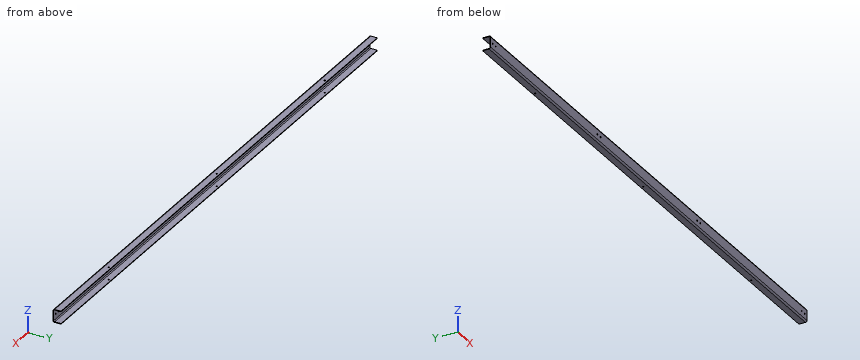
```python
from build123d import *

# Parameters (mm, degrees)
BASE_FLANGE1_DEPTH = 1928.8125
SKETCH2_R          = 2.4511
CUT_EXTRUDE1_DEPTH = 1930.51962345
SKETCH3_R          = 2.4511
CUT_EXTRUDE2_DEPTH = 1930.51962345
FILLET1_R          = 3.175


# Sheet-metal steps are written as plain solids
with BuildPart() as part:
    # Sketch1 → Base-Flange1 (new body)
    with BuildSketch(Plane(origin=(0, 0, 0), x_dir=(0, 0, -1), z_dir=(1, 0, 0))):
        with BuildLine():
            Line((0, 27.432), (0, 5.207))
            ThreePointArc((0, 5.207), (1.52509499, 1.52509499), (5.207, 0))
            Line((5.207, 0), (39.243, 0))
            ThreePointArc((39.243, 0), (42.92490501, 1.52509499), (44.45, 5.207))
            Line((44.45, 5.207), (44.45, 27.432))
            Line((44.45, 27.432), (42.418, 27.432))
            Line((42.418, 27.432), (42.418, 5.207))
            ThreePointArc((42.418, 5.207), (41.48806403, 2.96193597), (39.243, 2.032))
            Line((39.243, 2.032), (5.207, 2.032))
            ThreePointArc((5.207, 2.032), (2.96193597, 2.96193597), (2.032, 5.207))
            Line((2.032, 5.207), (2.032, 27.432))
            Line((2.032, 27.432), (0, 27.432))
        make_face()
    extrude(amount=BASE_FLANGE1_DEPTH)

    # Sketch2 → Cut-Extrude1 (cut, through all)
    with BuildSketch(Plane(origin=(0, 0, 0), x_dir=(-1, 0, 0), z_dir=(0, -1, 0))):
        with Locations(Location((-12.7, 22.225, 0), (0, 0, 90))):
            Circle(SKETCH2_R)
        with Locations(Location((-31.75, 22.225, 0), (0, 0, 90))):
            Circle(SKETCH2_R)
        with Locations(Location((-650.90675, 22.225, 0), (0, 0, 90))):
            Circle(SKETCH2_R)
        with Locations(Location((-669.95675, 22.225, 0), (0, 0, 90))):
            Circle(SKETCH2_R)
        with Locations(Location((-1916.1125, 22.225, 0), (0, 0, 270))):
            Circle(SKETCH2_R)
        with Locations(Location((-1897.0625, 22.225, 0), (0, 0, 270))):
            Circle(SKETCH2_R)
        with Locations(Location((-1277.90575, 22.225, 0), (0, 0, 270))):
            Circle(SKETCH2_R)
        with Locations(Location((-1258.85575, 22.225, 0), (0, 0, 270))):
            Circle(SKETCH2_R)
    extrude(amount=-CUT_EXTRUDE1_DEPTH, mode=Mode.SUBTRACT)

    # Sketch3 → Cut-Extrude2 (cut, through all)
    with BuildSketch(Plane(origin=(0, 0, -44.45), x_dir=(-1, 0, 0), z_dir=(0, 0, -1))):
        with Locations((-1623.21875, 19.05)):
            Circle(SKETCH3_R)
        with Locations((-964.40625, 19.05)):
            Circle(SKETCH3_R)
        with Locations((-305.59375, 19.05)):
            Circle(SKETCH3_R)
    extrude(amount=-CUT_EXTRUDE2_DEPTH, mode=Mode.SUBTRACT)

    # Fillet1
    fillet1_edges = [part.edges().sort_by_distance(p)[0] for p in [
        (0, 27.432, -1.016),
        (0, 27.432, -43.434),
        (1928.8125, 27.432, -1.016),
        (1928.8125, 27.432, -43.434),
    ]]
    fillet(fillet1_edges, radius=FILLET1_R)


solid = part.part
```
The listing builds one solid part. Answer for the finished solid, in the listing's coordinates (mm). Give positions to 0.01 mm unless a question says otherwise; leave off trailing zeros. Write each loop counter-clockwise with the first axis right and the second up, starting at its lowest first coordinate (ties: lowest second). Pieces come first, ordered by that corner, then holes. Notation, with made-up numbers: (72.5, 27) -> (125.5, 27) arc R28 ccw to (125.5, 61) -> close; hole circle Ø8 at (56, 37). An arc over 180 degrees is marked (long way). Use one line per item in the form item = value.
1) Section A-A on y = 11.25 is taken. Write down the section's boundary in (x, z).
Result:
outline = (0, -44.45) -> (1928.81, -44.45) -> (1928.81, -42.42) -> (0, -42.42) -> close; (0, -2.03) -> (1928.81, -2.03) -> (1928.81, 0) -> (0, 0) -> close
2) Each of these flat-tipped pins is pushed along its axis until it touches: P1, Ø6, axis at x = 475, z = -8.5, coming from the +Y side; P2, Ø4, axis at y = 4.5, z = -8.5, coming from the -X side. Where does it stop, or does it pass through?
Result:
P1 = 2.03
P2 = through
3) Section B-B on x = 1587 is taken. Write down the section's boundary in (y, z) (3 decimals).
Result:
outline = (0, -39.243) arc R5.207 ccw to (5.207, -44.45) -> (27.432, -44.45) -> (27.432, -42.418) -> (5.207, -42.418) arc R3.175 cw to (2.032, -39.243) -> (2.032, -5.207) arc R3.175 cw to (5.207, -2.032) -> (27.432, -2.032) -> (27.432, 0) -> (5.207, 0) arc R5.207 ccw to (0, -5.207) -> close
4) Straight lines are drawn through the part: probe 1 along Z at (x, y) = (1053, 24); probe 2 along Z at (x, y) = (1447, 4.25); probe 3 along Y at (x, z) = (930, -14.5). For each, find the intervals that lie inside material, in ascending order.
Result:
probe_1 = -44.45 to -42.42, -2.03 to 0
probe_2 = -44.36 to -42.27, -2.18 to -0.09
probe_3 = 0 to 2.03
